```python
from build123d import *

# Parameters (mm, degrees)
SKETCH1_W                                      = 19.98
SKETCH1_H                                      = 128.4
BOSS_EXTRUDE1_DEPTH                            = 2.5
CUT_EXTRUDE1_DEPTH                             = 127.049239982
CUT_EXTRUDE2_DEPTH                             = 127.049239982
SKETCH4_W                                      = 3.9
SKETCH4_H                                      = 14.6
CUT_EXTRUDE3_DEPTH                             = 127.049239982
F_3_0_3_DIAMETER_HOLE1_D                       = 3
CSK_FOR_M2_5_FLAT_HEAD_MACHINE_SCREW1_AT_COUNT = 2
CSK_FOR_M2_5_FLAT_HEAD_MACHINE_SCREW1_AT_PITCH = 99.130249672
USB_DEPTH                                      = 127.049239982
SKETCH10_R                                     = 2
LEDS_DEPTH                                     = 127.049239982
SKETCH11_R                                     = 2
SINGLE_LED_DEPTH                               = 127.049239982
SKETCH13_W                                     = 9
SKETCH13_H                                     = 6.5
DISABLE_COMMS_DEPTH                            = 127.049239982
SKETCH14_W                                     = 13.2
SKETCH14_H                                     = 17
RJ45_DEPTH                                     = 127.049239982
SKETCH15_W                                     = 10.8
SKETCH15_H                                     = 18
OUTPUT_DEPTH                                   = 127.049239982
SKETCH16_W                                     = 11.5
SKETCH16_H                                     = 10
POWER_DEPTH                                    = 127.049239982
FILLETS_R                                      = 0.5
FILLET2_R                                      = 0.5


with BuildPart() as part:
    # Sketch1 → Boss-Extrude1 (new body)
    with BuildSketch(Plane.XY.offset(2.5)):
        with Locations((2.54, 61.2)):
            Rectangle(SKETCH1_W, SKETCH1_H)
    extrude(amount=-BOSS_EXTRUDE1_DEPTH)

    # Sketch2 → Cut-Extrude1 (cut, through all)
    with BuildSketch(Plane.XY.offset(2.5)):
        with BuildLine():
            Line((2.445403852, 124.05), (-2.445403852, 124.05))
            ThreePointArc((-2.445403852, 124.05), (-2.95, 122.4), (-2.445403852, 120.75))
            Line((-2.445403852, 120.75), (2.445403852, 120.75))
            ThreePointArc((2.445403852, 120.75), (2.95, 122.4), (2.445403852, 124.05))
        make_face()
    extrude(amount=-CUT_EXTRUDE1_DEPTH, mode=Mode.SUBTRACT)

    # Sketch3 → Cut-Extrude2 (cut, through all)
    with BuildSketch(Plane.XY.offset(2.5)):
        with BuildLine():
            Line((7.525403852, 1.65), (2.634596148, 1.65))
            ThreePointArc((2.634596148, 1.65), (2.13, 0), (2.634596148, -1.65))
            Line((2.634596148, -1.65), (7.525403852, -1.65))
            ThreePointArc((7.525403852, -1.65), (8.03, 0), (7.525403852, 1.65))
        make_face()
    extrude(amount=-CUT_EXTRUDE2_DEPTH, mode=Mode.SUBTRACT)

    # Sketch4 → Cut-Extrude3 (cut, through all)
    with BuildSketch(Plane(origin=(0, 0, 0), x_dir=(-1, 0, 0), z_dir=(0, 0, -1))):
        with Locations((1.87, 8.5)):
            Rectangle(SKETCH4_W, SKETCH4_H)
    extrude(amount=-CUT_EXTRUDE3_DEPTH, mode=Mode.SUBTRACT)

    # Ø3.0 (3) Diameter Hole1 (through all)
    with Locations(Plane.XY.offset(2.5)):
        with Locations((-3.95, 119.1)):
            Hole(F_3_0_3_DIAMETER_HOLE1_D / 2)

    # Sketch7 → CSK for M2.5 Flat Head Machine Screw1 (revolve, cut)
    with BuildSketch(Plane(origin=(5.08, 11.7, 2.5), x_dir=(0, -1, 0), z_dir=(1, 0, 0))):
        Polygon((0, 0), (0, 2.5), (1.35, 2.5), (1.35, 1.5), (2.5, 0.35), (2.5, 0), align=None)
    csk_for_m2_5_flat_head_machine_screw1 = revolve(axis=Axis((5.08, 11.7, 8.85), (0, 0, -1)), mode=Mode.SUBTRACT)

    # CSK for M2.5 Flat Head Machine Screw1 at: CSK for M2.5 Flat Head Machine Screw1 ×2
    with Locations(*[Vector(-0.05124570972853528, 0.9986860754183062, 0) * (i * CSK_FOR_M2_5_FLAT_HEAD_MACHINE_SCREW1_AT_PITCH) for i in range(1, CSK_FOR_M2_5_FLAT_HEAD_MACHINE_SCREW1_AT_COUNT)]):
        add(csk_for_m2_5_flat_head_machine_screw1, mode=Mode.SUBTRACT)

    # Sketch9 → USB (cut, through all)
    with BuildSketch(Plane.XY.offset(2.5)):
        Polygon((-3.82, 19.95), (1.78, 19.95), (1.78, 32.45), (-3.82, 32.45), (-6.95, 32.45), (-6.95, 19.95), align=None)
    extrude(amount=-USB_DEPTH, mode=Mode.SUBTRACT)

    # Sketch10 → LEDs (cut, through all)
    with BuildSketch(Plane.XY.offset(2.5)):
        with Locations((-1.28, 34.72)):
            Circle(SKETCH10_R)
        with Locations((3.8, 34.72)):
            Circle(SKETCH10_R)
    extrude(amount=-LEDS_DEPTH, mode=Mode.SUBTRACT)

    # Sketch11 → Single LED (cut, through all)
    with BuildSketch(Plane.XY.offset(2.5)):
        with Locations((1.18, 42.62)):
            Circle(SKETCH11_R)
    extrude(amount=-SINGLE_LED_DEPTH, mode=Mode.SUBTRACT)

    # Sketch13 → Disable comms (cut, through all)
    with BuildSketch(Plane.XY.offset(2.5)):
        with Locations((0.505, 51.2)):
            Rectangle(SKETCH13_W, SKETCH13_H)
    extrude(amount=-DISABLE_COMMS_DEPTH, mode=Mode.SUBTRACT)

    # Sketch14 → RJ45 (cut, through all)
    with BuildSketch(Plane.XY.offset(2.5)):
        with Locations((2.78, 63.2)):
            Rectangle(SKETCH14_W, SKETCH14_H)
    extrude(amount=-RJ45_DEPTH, mode=Mode.SUBTRACT)

    # Sketch15 → Output (cut, through all)
    with BuildSketch(Plane.XY.offset(2.5)):
        with Locations((1.58, 81.2)):
            Rectangle(SKETCH15_W, SKETCH15_H)
    extrude(amount=-OUTPUT_DEPTH, mode=Mode.SUBTRACT)

    # Sketch16 → Power (cut, through all)
    with BuildSketch(Plane.XY.offset(2.5)):
        with Locations((1.93, 97.2)):
            Rectangle(SKETCH16_W, SKETCH16_H)
    extrude(amount=-POWER_DEPTH, mode=Mode.SUBTRACT)

    # Fillets
    fillets_edges = [part.edges().sort_by_distance(p)[0] for p in [
        (5.005, 54.45, 1.25),
        (5.005, 47.95, 1.25),
        (-3.995, 47.95, 1.25),
        (-3.995, 54.45, 1.25),
        (9.38, 54.7, 1.25),
        (-3.82, 54.7, 1.25),
        (-3.82, 71.7, 1.25),
        (9.38, 71.7, 1.25),
        (6.98, 72.2, 1.25),
        (-3.82, 72.2, 1.25),
        (-3.82, 90.2, 1.25),
        (6.98, 90.2, 1.25),
        (7.68, 92.2, 1.25),
        (-3.82, 92.2, 1.25),
        (-3.82, 102.2, 1.25),
        (7.68, 102.2, 1.25),
        (-3.82, 15.8, 1.25),
        (-3.82, 1.2, 1.25),
        (0.08, 1.2, 1.25),
        (0.08, 15.8, 1.25),
        (-6.95, 19.95, 1.25),
        (-6.95, 32.45, 1.25),
        (1.78, 32.45, 1.25),
        (1.78, 19.95, 1.25),
    ]]
    fillet(fillets_edges, radius=FILLETS_R)

    # Fillet2
    fillet2_edges = [part.edges().sort_by_distance(p)[0] for p in [
        (-7.45, 61.2, 0),
        (2.54, -3, 0),
        (12.53, 61.2, 0),
        (2.54, 125.4, 0),
    ]]
    fillet(fillet2_edges, radius=FILLET2_R - 0.0001)  # a hair under: the kernel refuses the full size


solid = part.part
```
Can you work these out from the model? Positions are in its coordinate system, mm. A direction names the side the tool comes from. Give positions to 0.01 mm unless a question says otherwise; leave off trailing zeros. Loops run counter-clockwise (first coordinate to the right, second up) from the corner with the lowest first, then second, coordinate; pieces in that order, holes last. Notation, with made-up numbers: M 11,-36 L 50,-36 A11 cw 50,-28 Z; hole C 6.25,81.5 d5. An arc over 180 degrees is marked long. One line per item, written item: value.
(1) Suppose I cut it at C-C on y = 42.62. List the corners of the cut face in (x, z) for me, plus the area to 3 significant figures.
Returned:
outline: M -7.45,0.5 A0.5 ccw -6.95,0 L -0.82,0 L -0.82,2.5 L -7.45,2.5 Z; M 3.18,0 L 12.03,0 A0.5 ccw 12.53,0.5 L 12.53,2.5 L 3.18,2.5 Z
area: 39.8 mm^2
(2) We'd pull the mould along X, two halves only. Please class faces 4 (the face through (2, -3, 2)), 5 (the face through (2.95, 122.38, 1.27)), 6 (the face through (12.53, 60, 2)): released by +X, released by -X, zero draft, split by the parting line, or undercut.
Returned:
face 4: zero draft
face 5: undercut
face 6: released by +X
(3) Which directions (+Z, -Z, +X, -X, +Y, -Y) give clear straight access to the entire face, cutting with the end or side of a thin tool? Please do faces 1 (the face through (5, 14.2, 2.3)), 2 (the face through (0.08, 8, 1)), 3 (the face through (-7.45, 60, 2)).
Returned:
face 1: +Z
face 2: +Z, -Z
face 3: +Z, -Z, -X, +Y, -Y
(4) Suppose I cut it at B-B on y = 61.5. List the corners of the cut face in (x, z) for me.
Returned:
outline: M -7.45,0.5 A0.5 ccw -6.95,0 L -3.82,0 L -3.82,2.5 L -7.45,2.5 Z; M 9.38,0 L 12.03,0 A0.5 ccw 12.53,0.5 L 12.53,2.5 L 9.38,2.5 Z
(5) I need wall thicknesses on line 1 (X direction, y = 11.7, z = 0.7); line 2 (X direction, y = 11.7, z = 2.3); line 3 (X direction, y = 52, z = 0.85) (3 decimals). Which ranges of each line are inside material? Lowest first, please.
Returned:
line 1: -7.45 to -3.82, 0.08 to 3.73, 6.43 to 12.53
line 2: -7.45 to -3.82, 0.08 to 2.58, 7.58 to 12.53
line 3: -7.45 to -3.995, 5.005 to 12.53
(6) Will this pin go through, and if not, where does the flat tip stop? pin 1 (4.5 mm diameter, centred on x = 0, y = 110.7, fed in from +Z).
Returned:
pin 1: z = 1.9
(7) Suppose I cut it at A-A on y = 11.7. List the corners of the cut face in (x, z) for me.
Returned:
outline: M -7.45,0.5 A0.5 ccw -6.95,0 L -3.82,0 L -3.82,2.5 L -7.45,2.5 Z; M 0.08,0 L 3.73,0 L 3.73,1 L 2.58,2.15 L 2.58,2.5 L 0.08,2.5 Z; M 6.43,0 L 12.03,0 A0.5 ccw 12.53,0.5 L 12.53,2.5 L 7.58,2.5 L 7.58,2.15 L 6.43,1 Z
